Verification items for this drawing (mm, ordinates from the low corner). Round coordinates to 2 decimals unless told otherwise and drop trailing zeros. Loops run counter-clockwise (first coordinate to the right, second up) from the corner with the lowest first, then second, coordinate; pieces in that order, holes last. Notation, with made-up numbers: (87.5, -8.75) - (110.5, -8.75) arc R32 ccw to (110.5, 20.25) - close; hole circle Ø10 at (15.25, -6). An arc over 180 degrees is marked (long way). Put each result on its own line as item: value. Start each with the question number.
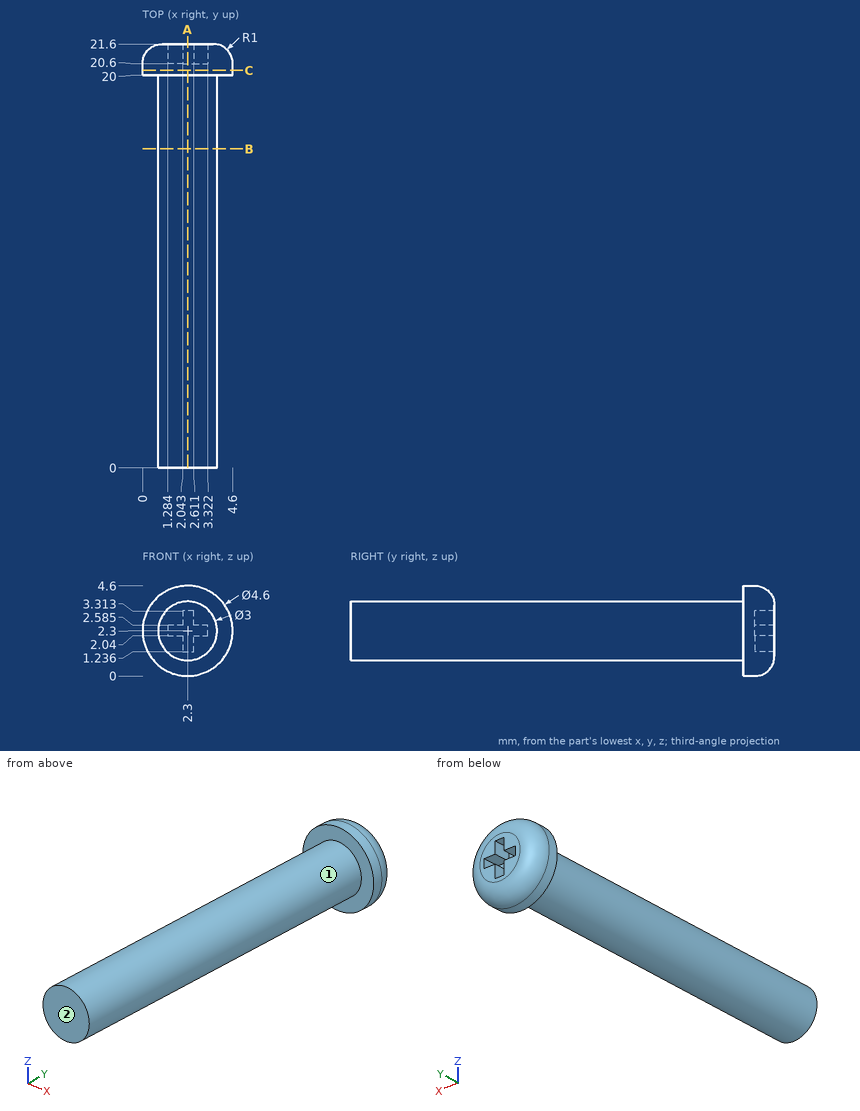
Q1. Cross-section at A-A on x = 2.3. Enter the section's corners in (y, z).
Q2. Draft check along Z on the marked faces 1 and 2. Enter one of: +Z half, -Z half, draft (parallel to the pull), parting line (faces both ways), or undercut.
Q3. Cross-section at C-C on y = 20.25. Enter the section's corners in (x, z), and give its area (3 significant figures).
Q4. Material ranges on line 1 (Y direction, x = 1.85, z = 3.6); line 2 (Z direction, x = 1.2, y = 2.5); line 3 (Z direction, x = 2.2, y = 15), recorded low to high. Write a range as from..to.
Q5. Cross-section at B-B on y = 16.25. Enter the section's corners in (x, z).
Q6. Depth check by flat-ended pin: pin 1 Ø0.6 at (x, y) = (1.5, 21) entering from -Z (1 decimal); pin 2 Ø1.5 at (y, z) = (4, 1) entering from +X (1 decimal); pin 3 Ø0.8 at (y, z) = (21, 3) entering from +X (1 decimal). Enter the tip coordinate at first touch or a pass-through.
Answer list:
1. outline: (0, 0.8) - (20, 0.8) - (20, 0) - (20.6, 0) arc R1 ccw to (21.6, 1) - (21.6, 1.24) - (20.6, 1.24) - (20.6, 3.31) - (21.6, 3.31) - (21.6, 3.6) arc R1 ccw to (20.6, 4.6) - (20, 4.6) - (20, 3.8) - (0, 3.8) - close
2. face 1: parting line
2. face 2: draft
3. outline: circle Ø4.6 at (2.3, 2.3)
3. area: 16.6 mm2
4. line 1: y = 0..21.6
4. line 2: z = 1.28..3.32
4. line 3: z = 0.8..3.8
5. outline: circle Ø3 at (2.3, 2.3)
6. pin 1: stops at z = 0.1
6. pin 2: stops at x = 3.7
6. pin 3: stops at x = 4.6
